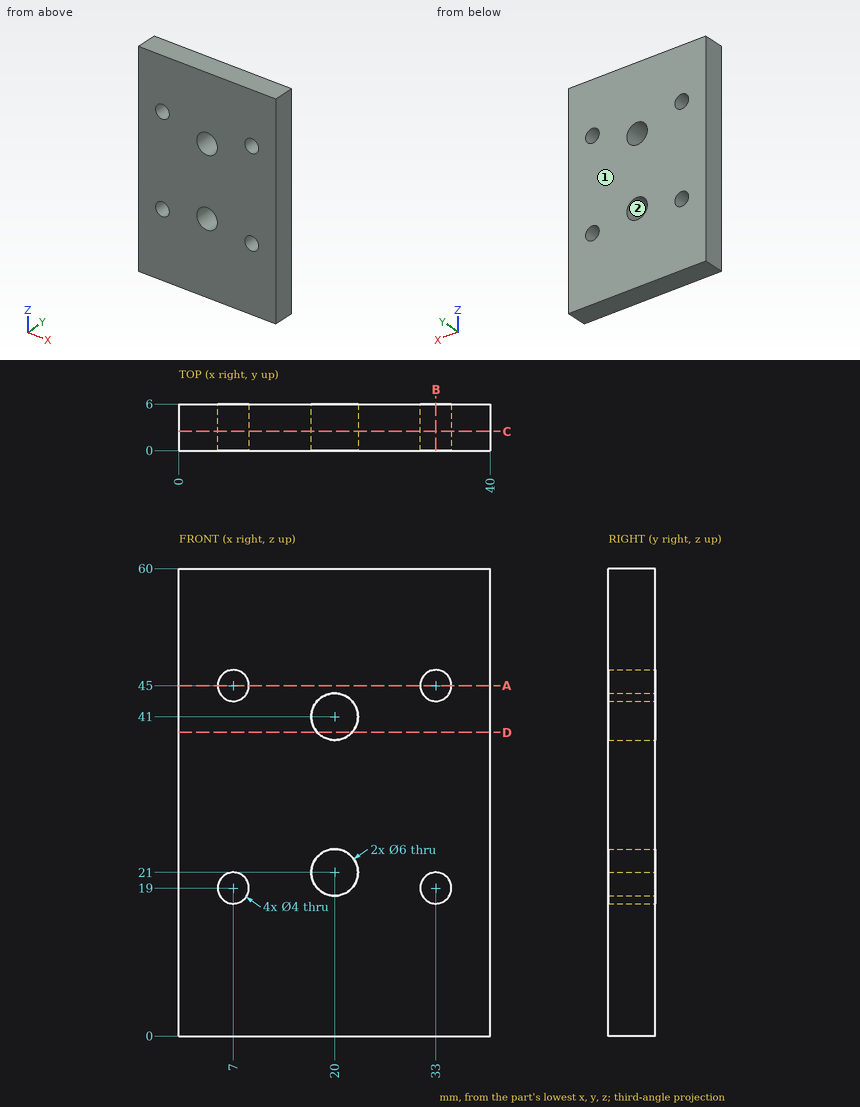
The figure shows three views and two pictorial views of one solid part (mm, origin at its lowest corner). Answer the questions. Coordinates: 2 decimals unless noted, no trailing zeros. Loops run counter-clockwise (first coordinate to the right, second up) from the corner with the lowest first, then second, coordinate; pieces in that order, holes last.
(1) The part is cut by section B-B (x = 33). Determine the outline of the cut face in (y, z), and give its area (3 significant figures).
Solution:
outline: (0, 0) - (6, 0) - (6, 17) - (0, 17) - close; (0, 21) - (6, 21) - (6, 43) - (0, 43) - close; (0, 47) - (6, 47) - (6, 60) - (0, 60) - close
area: 312 mm2
(2) Consider line 1 along Z through (x, y) = (33, 3.95); line 2 along X through (y, z) = (4.5, 46.5); line 3 along Z through (x, y) = (19, 4.25). Determine where each line is inside the solid, lowest interval first.
Solution:
line 1: z = 0 to 17, 21 to 43, 47 to 60
line 2: x = 0 to 5.68, 8.32 to 31.68, 34.32 to 40
line 3: z = 0 to 18.17, 23.83 to 38.17, 43.83 to 60
(3) Flat-ended cylindrical pins translate along their axes: pin 1 Ø3.5 at (x, z) = (20, 41) entering from +Y; pin 2 Ø4.5 at (x, z) = (33, 19) entering from -Y. Find the tip coordinate at first contact, or state that the pin passes through.
Solution:
pin 1: passes through
pin 2: stops at y = 0
(4) The part is cut by section C-C (y = 2.5). Determine the outline of the cut face in (x, z).
Solution:
outline: (0, 0) - (40, 0) - (40, 60) - (0, 60) - close; hole circle Ø4 at (7, 19); hole circle Ø4 at (7, 45); hole circle Ø6 at (20, 21); hole circle Ø6 at (20, 41); hole circle Ø4 at (33, 19); hole circle Ø4 at (33, 45)
(5) The mould has two halves that part along X. Classify the marked faces 1 and 2: released by +X, released by -X, zero draft, split by the parting line, or undercut.
Solution:
face 1: zero draft
face 2: undercut
(6) The part is cut by section D-D (z = 39). Determine the outline of the cut face in (x, y).
Solution:
outline: (0, 0) - (17.76, 0) - (17.76, 6) - (0, 6) - close; (22.24, 0) - (40, 0) - (40, 6) - (22.24, 6) - close
(7) The part is cut by section A-A (z = 45). Determine the outline of the cut face in (x, y).
Solution:
outline: (0, 0) - (5, 0) - (5, 6) - (0, 6) - close; (9, 0) - (31, 0) - (31, 6) - (9, 6) - close; (35, 0) - (40, 0) - (40, 6) - (35, 6) - close
